Autodesk Inventor part; units mm, degrees
ref_plane "YZ Plane" through (0, 0, 0) normal (1, 0, 0) x (0, 1, 0)
ref_plane "XZ Plane" through (0, 0, 0) normal (0, 1, 0) x (-1, 0, 0)
ref_plane "XY Plane" through (0, 0, 0) normal (0, 0, 1) x (1, 0, 0)
sketch "Sketch1" plane through (0, 0, 0) normal (0, 1, 0) x (-1, 0, 0)
  line L0 (0, 0) -> (13.97, 0)
  line L1 (13.97, 0) -> (13.97, -15.748)
  line L2 (13.97, -15.748) -> (0, -15.748)
  line L3 (0, -15.748) -> (0, 0)
  line L4 (13.97, -49.53) -> (0, -49.53)
  line L5 (0, -49.53) -> (0, -65.278)
  line L6 (0, -65.278) -> (13.97, -65.278)
  line L7 (13.97, -65.278) -> (13.97, -49.53)
  dimension "d0" = 13.97
  dimension "d1" = 15.748
  dimension "d2" = 15.748
  dimension "d3" = 33.782
extrude "Extrusion1" add sketch "Sketch1" along normal blind 2.286
sketch "Sketch2" plane through (0, 2.286, 0) normal (0, 1, 0) x (1, 0, 0)
  line L0 (-13.97, 15.748) -> (-13.97, 0)
  line L1 (-13.97, 0) -> (0, 0)
  line L2 (0, 0) -> (0, 65.278)
  line L3 (0, 65.278) -> (-13.97, 65.278)
  line L4 (-13.97, 65.278) -> (-13.97, 0)
  point P0 (0, 0)
extrude "Extrusion2" add sketch "Sketch2" along normal blind 6.35
sketch "Sketch3" plane through (0, 0, -49.53) normal (1, 0, 0) x (0, 0, -1)
  line L0 (-49.53, 8.636) -> (15.748, 8.636)
  line L1 (15.748, 0) -> (15.748, 8.636)
  line L2 (-49.53, 8.636) -> (15.748, 8.636)
  line L3 (15.748, 8.636) -> (15.748, 2.5059)
  line L4 (15.748, 2.5059) -> (-49.53, 2.5059)
  line L5 (-49.53, 2.5059) -> (-49.53, 8.636)
  point P0 (-49.53, 0)
extrude "Extrusion3" add sketch "Sketch3" along normal blind 12.446
sketch "Sketch4" plane through (12.446, 0, -49.53) normal (1, 0, 0) x (0, 0, -1)
  line L0 (15.748, 8.636) -> (-49.53, 8.636)
  line L1 (-49.53, 8.636) -> (15.748, 8.636)
  line L2 (15.748, 8.636) -> (15.748, 2.5059)
  line L3 (15.748, 2.5059) -> (-49.53, 2.5059)
  line L4 (-49.53, 0) -> (-49.53, 8.636)
  line L5 (-49.53, 8.636) -> (-49.53, 2.5059)
  line L6 (-49.53, 2.5059) -> (-24.0466, 2.5059) construction
  line L7 (-16.891, 8.636) -> (-16.891, -118.364) construction
  line L8 (15.748, 2.5059) -> (-49.53, 2.5059)
  line L9 (-49.53, 2.5059) -> (-16.891, -30.1331)
  line L10 (-49.53, 2.5059) -> (-3.3715, 2.5059) construction
  line L11 (-16.891, -30.1331) -> (15.748, 2.5059)
  line L12 (-33.2105, -13.8136) -> (-0.5715, -13.8136)
  line L13 (-16.891, -8.7336) -> (-2.6757, -8.7336)
  line L14 (-49.53, 2.5059) -> (15.748, 2.5059)
  line L15 (-2.6757, -8.7336) -> (3.4838, -2.5741)
  line L16 (3.4838, -2.5741) -> (-36.2655, -2.5741)
  line L17 (-30.106, -8.7336) -> (-16.891, -8.7336)
  line L18 (-16.891, -8.7336) -> (-31.1063, -8.7336)
  line L19 (-31.1063, -8.7336) -> (-37.2658, -2.5741)
  line L20 (-37.2658, -2.5741) -> (2.4835, -2.5741)
  point P0 (-30.106, -8.7336)
  point P1 (-36.2655, -2.5741)
  dimension "d13" = 127
  dimension "d14" = 45
  dimension "d15" = 5.08
  dimension "d16" = 5.08
  dimension "d17" = 5.08
extrude "Extrusion4" add sketch "Sketch4" along normal blind 6.35 contours L2 L3 L4 L0 | L11 L12 L9 L3
sketch "Sketch5" plane through (18.796, 0, -49.53) normal (1, 0, 0) x (0, 0, -1)
  line L0 (-33.2105, -13.8136) -> (-0.5715, -13.8136)
  line L1 (-33.2105, -13.8136) -> (-0.5715, -13.8136)
  line L2 (-0.5715, -13.8136) -> (-0.5715, -8.8161)
  line L3 (-0.5715, -8.8161) -> (-33.2105, -8.8161)
  line L4 (-33.2105, -8.8161) -> (-33.2105, -13.8136)
  point P0 (-49.53, 0)
ref_plane "Work Plane1" through (-13.97, 0, -32.639) normal (0, 0, 1) x (1, 0, 0)
sketch "Sketch6" plane through (-13.97, 0, -32.639) normal (0, 0, 1) x (1, 0, 0)
  line L0 (26.416, -8.7336) -> (32.766, -8.7336)
  line L1 (32.766, -8.7336) -> (41.9683, -8.7336)
  line L2 (41.9683, -8.7336) -> (44.4776, -6.1913)
  line L3 (44.4776, -6.1913) -> (47.7281, -9.3996)
  line L4 (47.7281, -9.3996) -> (44.4776, -12.6928)
  line L5 (44.4776, -12.6928) -> (32.766, -12.6928)
  line L6 (32.766, -8.7336) -> (32.766, -12.6928)
  line L7 (32.766, 2.5059) -> (32.766, -13.8136)
  point P0 (13.97, 0)
extrude "Extrusion5" add sketch "Sketch6" along normal mid plane 28.575
sketch "Sketch7" plane through (0, 0, 0) normal (0, -1, 0) x (1, 0, 0)
  line L0 (0, -65.278) -> (0, 0)
  line L1 (0, -65.278) -> (-22.225, -65.278)
  line L2 (-22.225, -65.278) -> (-22.225, -49.53)
  line L3 (-22.225, -49.53) -> (0, -49.53)
  line L4 (0, -49.53) -> (0, -65.278)
  line L5 (-13.97, -65.278) -> (-13.97, 0) construction
  line L6 (-13.97, -32.639) -> (9.5461, -32.639) construction
  line L7 (0, 0) -> (0, -65.278)
  line L8 (0, 0) -> (-22.225, 0)
  line L9 (-22.225, 0) -> (-22.225, -15.748)
  line L10 (-22.225, -15.748) -> (0, -15.748)
  point P0 (0, -49.53)
  point P1 (0, -15.748)
  dimension "d24" = 22.225
extrude "Extrusion6" add sketch "Sketch7" along normal blind 6.35
chamfer "Chamfer1" distance 3.175 angle 45 2 edges at (0, -6.35, -7.874) (0, -6.35, -57.404)
chamfer "Chamfer2" distance 1.0795 angle 45 1 edges at (18.796, -12.6928, -32.639)
properties part number "FRC Pit Hook"
CAD build for the part. Positions are in the model's coordinates, mm. A direction names the side the tool comes from. Give positions to 0.01 mm unless a question says otherwise; leave off trailing zeros. Order: outer loops, then holes, each group sorted by start corner. A loop starts at its lowest first (then second) coordinate and runs counter-clockwise, first axis right, second up.
(1) Saw through at D-D, the plane y = -0.75. Give the cut face in (x, z) (3 decimals).
(2) Saw through at B-B, the plane x = 17.5. Give the cut face in (y, z).
(3) Saw through at C-C, the plane y = -5.25. Give the cut face in (x, z) (3 decimals).
(4) Mould opens along Z. For faces 5 (the flat face through (15.58, -5.7, -15.39)), 6 (the flat face through (15.58, -5.7, -49.89)), 7 (the flat face through (15.58, -5.77, -57)), 8 (the flat face through (-18, 0, -8)) say: released by +Z, released by -Z, zero draft, split by the parting line, or undercut.
(5) Tool access for faces 1 (the flat face through (-13, -6.35, -8)), 2 (the flat face through (12.446, -2, -32)), 3 (the flat face through (25, -12.693, -33)), 4 (the flat face through (26, -11, -46.926)): list every direction of +Z, -Z, +X, -X, +Y, -Y with a clear straight run to the whole face (end or side of a thin tool).
(6) Drill centre lines: L1, parallel to X at y = -2.25, z = -15 (3 decimals); L2, parallel to Z at x = -2.5, y = -4.5; L3, parallel to X at y = 0.75, z = -53. Where is each one in solid material? Low to high.
(7) Saw through at A-A, the plane z = -24. Give the cut face in (x, y).
(8) Flat gauge pins, fed straight in: pin 1 (5 mm diameter, centred on y = -5.5, z = -24, fed in from -X); pin 2 (4 mm diameter, centred on x = -17, z = -58.5, fed in from +Y); pin 3 (8 mm diameter, centred on x = 20.5, z = -48.5, fed in from -Y); pin 4 (1.5 mm diameter, centred on x = 27.5, y = -7.5, fed in from +Z). Where does each tip first touch, or does it go through?
Results found:
1. outline: (-22.225, -65.278) - (0, -65.278) - (0, -49.53) - (-22.225, -49.53) - close; (-22.225, -15.748) - (0, -15.748) - (0, 0) - (-22.225, 0) - close; (12.446, -62.022) - (18.796, -62.022) - (18.796, -3.256) - (12.446, -3.256) - close
2. outline: (-13.81, -48.96) - (2.51, -65.28) - (8.64, -65.28) - (8.64, 0) - (2.51, 0) - (-13.81, -16.32) - close; hole (-8.73, -46.85) - (-2.57, -53.01) - (-2.57, -12.26) - (-8.73, -18.42) - close
3. outline: (-22.225, -65.278) - (-2.075, -65.278) - (-2.075, -49.53) - (-22.225, -49.53) - close; (-22.225, -15.748) - (-2.075, -15.748) - (-2.075, 0) - (-22.225, 0) - close; (12.446, -57.522) - (18.796, -57.522) - (18.796, -50.338) - (12.446, -50.338) - close; (12.446, -14.94) - (18.796, -14.94) - (18.796, -7.756) - (12.446, -7.756) - close
4. face 5: undercut
4. face 6: undercut
4. face 7: released by -Z
4. face 8: zero draft
5. face 1: +Z, -Z, -X, -Y
5. face 2: +Z, -Z, -Y
5. face 3: +Z, -Z, +X, -Y
5. face 4: -Z, +X, +Y, -Y
6. L1: x = -22.225 to 0, 12.446 to 18.796
6. L2: z = -65.28 to -49.53, -15.75 to 0
6. L3: x = -13.97 to 0, 12.45 to 18.8
7. outline: (-13.97, 2.29) - (0, 2.29) - (0, 2.51) - (12.45, 2.51) - (12.45, -2.57) - (18.8, -2.57) - (18.8, 8.64) - (-13.97, 8.64) - close; (12.45, -13.81) - (18.8, -13.81) - (18.8, -13.77) - (19.88, -12.69) - (30.51, -12.69) - (33.76, -9.4) - (30.51, -6.19) - (28, -8.73) - (12.45, -8.73) - close
8. pin 1: stops at x = 28.72
8. pin 2: stops at y = 0
8. pin 3: stops at y = -13.81
8. pin 4: passes through
